Job drawing, mm, ordinate dimensions from the low corner. One solid piece. A direction names the side the tool comes from. Round coordinates to 2 decimals unless told otherwise and drop trailing zeros.
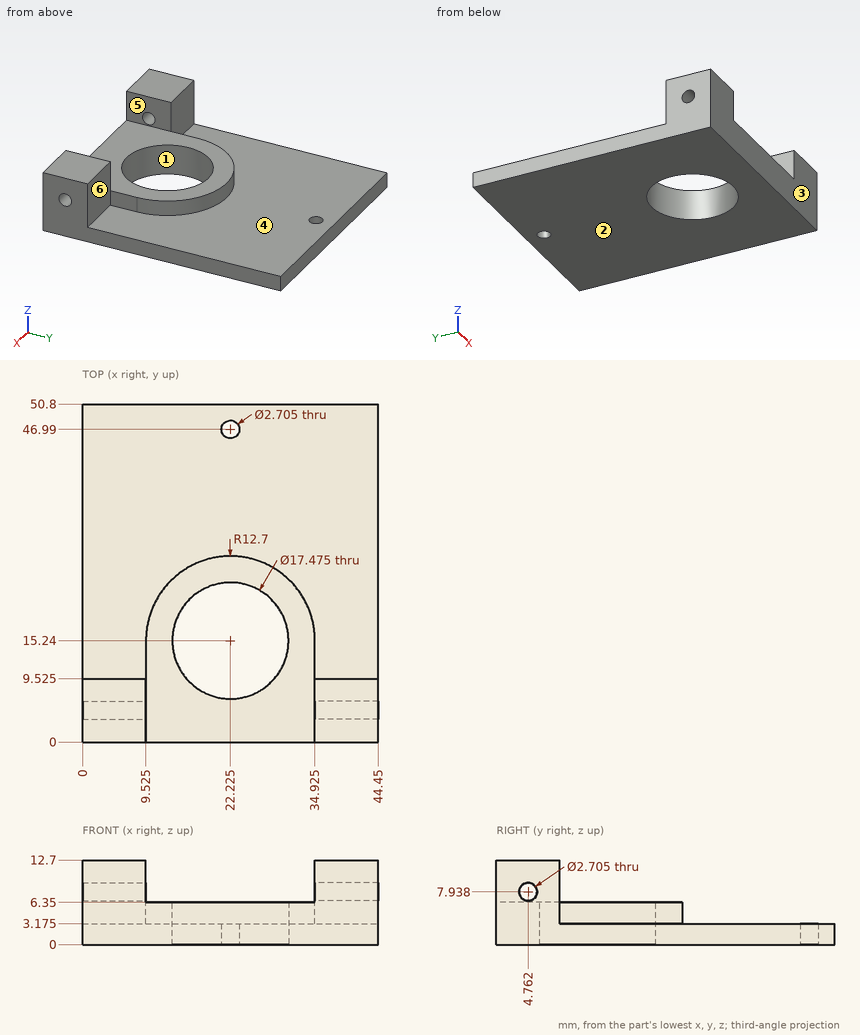
1) Tool access for the marked faces 4, 5 and 6: list every direction of +Z, -Z, +X, -X, +Y, -Y with a clear straight run to the whole face (end or side of a thin tool).
Values:
face 4: +Z, +Y
face 5: +Z, +Y, -Y
face 6: +Z, +X, +Y
2) Wall check: line 1 along X through (y, z) = (46.99, 1.7); line 2 along X through (y, z) = (11.5, 3.5) (1 decimal); line 3 along Z through (x, y) = (12, 22). Give the ranges that are in metal, low to high.
Values:
line 1: x = 0 to 20.87, 23.58 to 44.45
line 2: x = 9.5 to 14.3, 30.1 to 34.9
line 3: z = 0 to 6.35
3) Mould opens along Y. For the marked faces 1, 2 and 3 say: released by +Y, released by -Y, zero draft, split by the parting line, or undercut.
Values:
face 1: undercut
face 2: zero draft
face 3: released by -Y
4) Drop flat-ended pins along their axis: pin 1 Ø6 at (y, z) = (31, 7.5) entering from -X; pin 2 Ø12.5 at (x, y) = (21.5, 9.5) entering from +Z; pin 3 Ø4 at (x, y) = (11, 13.5) entering from -Z; pin 4 Ø4.5 at (x, y) = (22.225, 46.99) entering from +Z (1 decimal). Give the stop position or say it passes through.
Values:
pin 1: passes through
pin 2: stops at z = 6.35
pin 3: stops at z = 0
pin 4: stops at z = 3.2
